Answer from the drawing. Dimensions are ordinates in mm from the lowest x, y and z of the part. A direction names the side the tool comes from. Coordinates: 2 decimals unless noted, no trailing zeros. Write each loop counter-clockwise with the first axis right and the second up, starting at its lowest first coordinate (ties: lowest second). Pieces come first, ordered by that corner, then holes.
(1) Which of the six approach directions +Z, -Z, +X, -X, +Y, -Y give full straight-line access (tool end or side, diameter ignored) to the marked faces 4 and 5?
(2) Given P1, Ø3, axis at y = 5.5, z = 4, coming from the +X side; P2, Ø4, axis at x = 19, y = 11, coming from the +Z side; P3, Ø2.5, axis at x = 11, z = 7, coming from the -Y side; P4, Ø1, axis at x = 15, z = 10.5, coming from the +Y side, each flat-ended and moving along its own axis, determine where each tip first touches the part or whether it passes through.
(3) The part is cut by section B-B on y = 11. Determine the outline of the cut face in (x, z), plus the area to 3 significant figures.
(4) Straight lines are drawn through the part: line 1 (Y direction, x = 11, z = 0.85); line 2 (Z direction, x = 11, y = 14.65); line 3 (Z direction, x = 4, y = 3.5). For each, find the intervals that lie inside material, in ascending order.
(5) The part is cut by section A-A on x = 11. Determine the outline of the cut face in (y, z).
(6) The part is cut by section D-D on x = 19. Determine the outline of the cut face in (y, z).
(7) The part is cut by section C-C on z = 1.5. Determine the outline of the cut face in (x, y).
(8) For a pull along X with two mould halves and no side action, classify the marked faces 1, 2 and 3 as +X half, -X half, draft (parallel to the pull), parting line (faces both ways), or undercut.
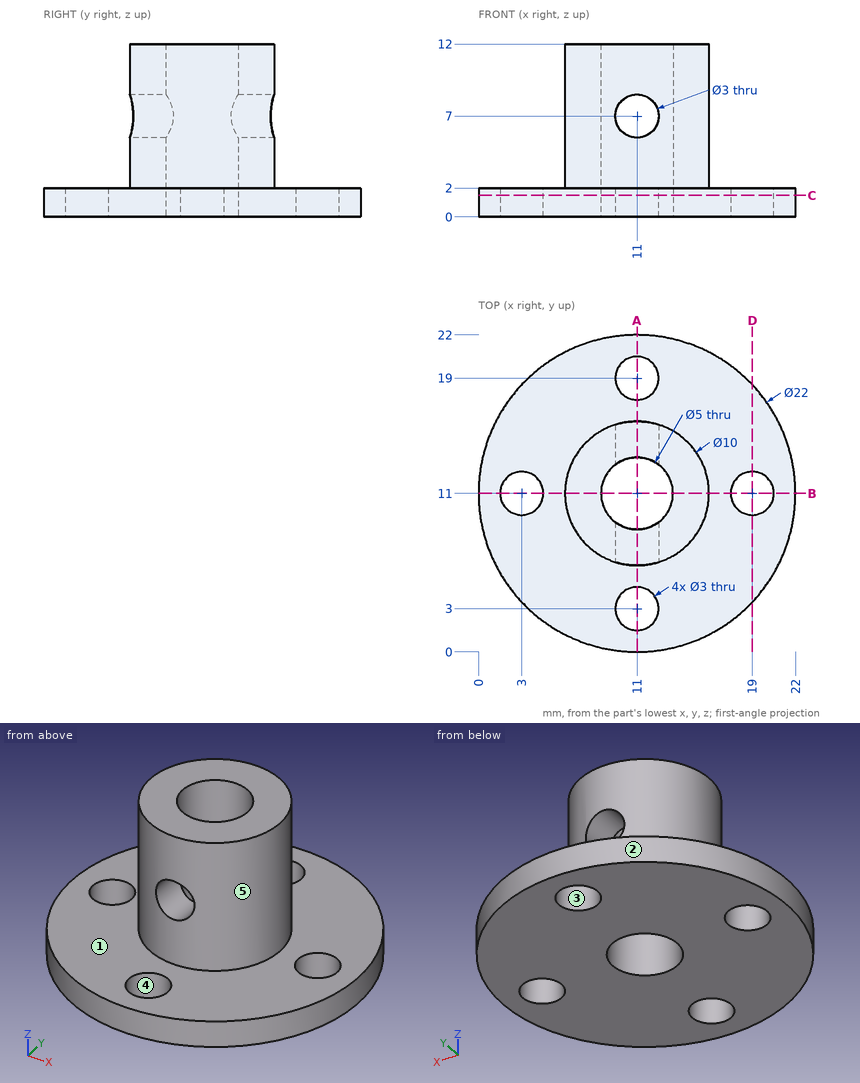
Model answer:
1. face 4: +Z, -Z
1. face 5: +Z
2. P1: stops at x = 14
2. P2: stops at z = 2
2. P3: passes through
2. P4: stops at y = 14.57
3. outline: (0, 0) - (1.5, 0) - (1.5, 2) - (0, 2) - close; (4.5, 0) - (8.5, 0) - (8.5, 12) - (6, 12) - (6, 2) - (4.5, 2) - close; (13.5, 0) - (17.5, 0) - (17.5, 2) - (16, 2) - (16, 12) - (13.5, 12) - close; (20.5, 0) - (22, 0) - (22, 2) - (20.5, 2) - close
3. area: 72.0 mm2
4. line 1: y = 0 to 1.5, 4.5 to 8.5, 13.5 to 17.5, 20.5 to 22
4. line 2: z = 0 to 5.5, 8.5 to 12
4. line 3: z = 0 to 2
5. outline: (0, 0) - (1.5, 0) - (1.5, 2) - (0, 2) - close; (4.5, 0) - (8.5, 0) - (8.5, 5.5) - (6, 5.5) - (6, 2) - (4.5, 2) - close; (6, 8.5) - (8.5, 8.5) - (8.5, 12) - (6, 12) - close; (13.5, 0) - (17.5, 0) - (17.5, 2) - (16, 2) - (16, 5.5) - (13.5, 5.5) - close; (13.5, 8.5) - (16, 8.5) - (16, 12) - (13.5, 12) - close; (20.5, 0) - (22, 0) - (22, 2) - (20.5, 2) - close
6. outline: (3.45, 0) - (9.5, 0) - (9.5, 2) - (3.45, 2) - close; (12.5, 0) - (18.55, 0) - (18.55, 2) - (12.5, 2) - close
7. outline: circle Ø22 at (11, 11); hole circle Ø3 at (3, 11); hole circle Ø5 at (11, 11); hole circle Ø3 at (11, 3); hole circle Ø3 at (11, 19); hole circle Ø3 at (19, 11)
8. face 1: draft
8. face 2: parting line
8. face 3: undercut
